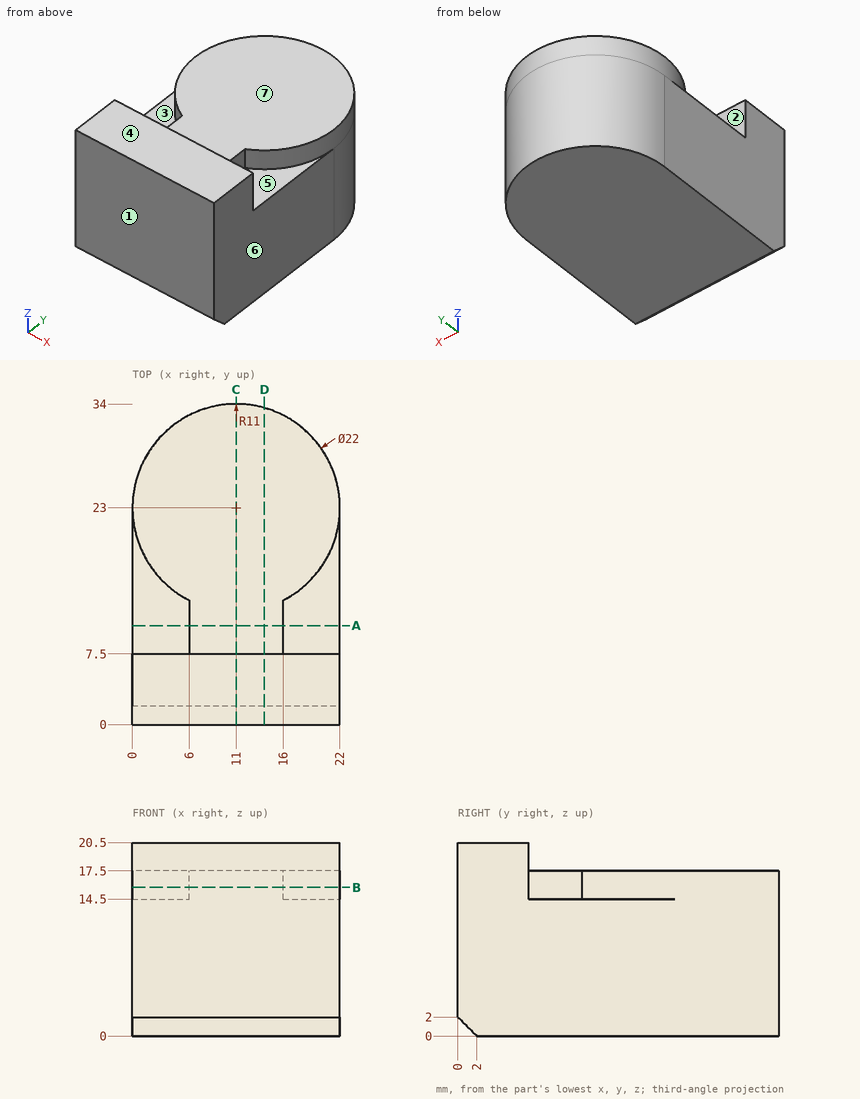
Geometry: see drawing. Coordinates: mm, zero at the bounding-box minimum. A direction names the side the tool comes from. Give positions to 0.01 mm unless a question says otherwise; leave off trailing zeros. Write each loop counter-clockwise with the first axis right and the second up, starting at its lowest first coordinate (ties: lowest second). Pieces come first, ordered by that corner, then holes. Notation, with made-up numbers: (-38, -28.75) - (4, -28.75) arc R35 ccw to (4, 5.25) - close; hole circle Ø9 at (42, 50.5). An arc over 180 degrees is marked (long way). Return JSON: item names as keys, results as strings. Group by question number.
1) Section D-D on x = 14. Return the cut outline in (y, z).
2) Section A-A on y = 10.5. Return the cut outline in (x, z).
3) Section B-B on z = 15.75. Return the cut outline in (x, y).
4) Section C-C on x = 11. Return the cut outline in (y, z), plus the area to 4 significant figures.
5) Mould query, pull axis Y, two halves, no side actions, for the marked faces 1, 2, 3 and 4. Classes: released by +Y, released by -Y, zero draft, split by the parting line, or undercut.
6) Line query: line 1 (Z direction, x = 12, y = 11.5); line 2 (Y direction, x = 1.75, z = 15.25); line 3 (Y direction, x = 17.25, z = 15.5). Output: solid intervals per line, ascending.
7) First-contact query: P1, Ø10, axis at x = 16, y = 28, coming from the -Z side; P2, Ø0.9, axis at y = 9, z = 15.5, coming from the -X side; P3, Ø3, axis at x = 8, z = 18.5, coming from the +Y side; P4, Ø3, axis at x = 3, y = 12.5, coming from the +Z side. Flat tips, straight axial feed; report the tip coordinate or a pass-through.
8) Set-up query: the marked faces 5, 6 and 7. Return all of +Z, -Z, +X, -X, +Y, -Y with unobstructed straight access to the full face (end or side cutting, diameter ignored); none if empty.
Filled in:
{
 "1": {"outline": "(0, 2) - (2, 0) - (33.58, 0) - (33.58, 17.5) - (7.5, 17.5) - (7.5, 20.5) - (0, 20.5) - close"},
 "2": {"outline": "(0, 0) - (22, 0) - (22, 14.5) - (16, 14.5) - (16, 17.5) - (6, 17.5) - (6, 14.5) - (0, 14.5) - close"},
 "3": {"outline": "(0, 0) - (22, 0) - (22, 7.5) - (16, 7.5) - (16, 13.2) arc R11 ccw (long way) to (6, 13.2) - (6, 7.5) - (0, 7.5) - close"},
 "4": {"outline": "(0, 2) - (2, 0) - (34, 0) - (34, 17.5) - (7.5, 17.5) - (7.5, 20.5) - (0, 20.5) - close", "area": "615.5 mm^2"},
 "5": {"face 1": "released by -Y", "face 2": "undercut", "face 3": "undercut", "face 4": "zero draft"},
 "6": {"line 1": "z = 0 to 17.5", "line 2": "y = 0 to 7.5, 17.05 to 28.95", "line 3": "y = 0 to 7.5, 13.95 to 32.05"},
 "7": {"P1": "stops at z = 0", "P2": "stops at x = 6", "P3": "stops at y = 33.84", "P4": "stops at z = 14.5"},
 "8": {"face 5": "+Z, +X", "face 6": "+Z, -Z, +X, +Y, -Y", "face 7": "+Z, +X, -X, +Y"}
}
